Verification items for the finished model (mm, model axes). A direction names the side the tool comes from. Round coordinates to 2 decimals unless told otherwise and drop trailing zeros. Order: outer loops, then holes, each group sorted by start corner. A loop starts at its lowest first (then second) coordinate and runs counter-clockwise, first axis right, second up. Notation, with made-up numbers: (36, -21) -> (49, -21) arc R23 ccw to (49, -5) -> close; hole circle Ø7 at (-4.5, 39). An arc over 180 degrees is marked (long way). Return JSON: item names as keys, results as strings. Group by question number.
1) Draft check along Y on faces 1 (the cylindrical face through (64.305, 26.799, -2.273)), 2 (the flat face through (32, 7, -12)), 3 (the cylindrical face through (64.305, 48.012, -23.486)), 4 (the flat face through (78, 36, -11)). Enter one of: pulls with the +Y half, pulls with the -Y half, needs draft (parallel to the pull), parting line crosses it, or undercut.
2) Scan lines: L1, parallel to Z at x = 29, y = 33.5 (3 decimals); L2, parallel to Z at x = 29, y = 18 (3 decimals); L3, parallel to X at y = 18, z = 12.25 (3 decimals). Record each from-to range of solid material in increasing order.
3) Tool access check on faces 5 (the flat face through (51, 60, -35)), 6 (the cylindrical face through (32.5, 33.13, -44.32)). Record the directions out of +Z, -Z, +X, -X, +Y, -Y that give a thin tool (end or side, any length) a straight path to the whole face; none if there is none.
4) Section check A-A on y = 11. Enter the section's corners in (x, z) (3 decimals), plus the area to 3 significant figures.
5) Section check C-C on y = 23. State how many separate pieces and enclosed holes the cut face has, plus the area to 3 significant figures.
6) Depth check by flat-ended pin: pin 1 (6 mm diameter, centred on x = 40, y = 31, fed in from +Z); pin 2 (5 mm diameter, centred on x = 29, z = -35.75, fed in from -Y); pin 3 (5 mm diameter, centred on x = 60.5, z = -8.5, fed in from -Y); pin 4 (8 mm diameter, centred on y = 32, z = -37, fed in from +X). Enter the tip coordinate at first touch or a pass-through.
Solid Edge part; units mm, degrees
sketch "Sketch1" plane through (0, 0, 0) normal (0, -1, 0) x (1, 0, 0)
  line L0 (-34, -45.75) -> (34, -45.75)
  line L1 (34, -45.75) -> (34, 45.75)
  line L2 (34, 45.75) -> (-34, 45.75)
  line L3 (-34, 45.75) -> (-34, -45.75)
  dimension "D1" = 34
  dimension "D2" = 34
extrude "Protrusion1" add sketch "Sketch1" against normal blind 12
sketch "Sketch2" plane through (0, 0, 0) normal (0, -1, 0) x (1, 0, 0)
  circle A0 centre (0, -14.75) radius 11.25
  circle A1 centre (-15.5, 0.75) radius 1.7
  circle A2 centre (-15.5, -30.25) radius 1.7
  circle A3 centre (15.5, -30.25) radius 1.7
  circle A4 centre (15.5, 0.75) radius 1.7
extrude "Cutout1" cut sketch "Sketch2" against normal through all
sketch "Sketch3" plane through (0, 0, 0) normal (0, -1, 0) x (1, 0, 0)
  circle A0 centre (7.7782, 36.0282) radius 1.4
  circle A1 centre (7.7782, 20.4718) radius 1.4
  circle A2 centre (-7.7782, 20.4718) radius 1.4
  circle A3 centre (-7.7782, 36.0282) radius 1.4
  circle A4 centre (0, 28.25) radius 6
  dimension "D1" = 7.7782
extrude "Cutout2" cut sketch "Sketch3" against normal through all
sketch "Sketch4" plane through (-34, 6, 0) normal (-1, 0, 0) x (0, 0, -1)
  line L0 (-19.89, -6) -> (45.75, -71.64)
  line L1 (45.75, -71.64) -> (45.75, -6)
  line L2 (45.75, -6) -> (-19.89, -6)
extrude "Extrusionsausprägung_2" add sketch "Sketch4" against normal blind 10
mirror "Mirror1" about plane through (0, 0, 0) normal (1, 0, 0) of "Extrusionsausprägung_2"
sketch "Sketch5" plane through (-34, 38.82, 0) normal (-1, 0, 0) x (0, 0, -1)
  circle A0 centre (33.7465, 1.4635) radius 1.875
  circle A1 centre (19.6043, 15.6057) radius 1.875
  dimension "D1" = 19.6043
extrude "Extrusionsausschnitt_3" cut sketch "Sketch5" against normal blind 14
sketch "Sketch6" plane through (-34, 38.82, 0) normal (-1, 0, 0) x (0, 0, -1)
  line L0 (45.75, -38.82) -> (-31.89, 38.82)
  line L1 (-31.89, 38.82) -> (-17.75, 38.82)
  line L2 (-17.75, 38.82) -> (45.75, -24.68)
  line L3 (45.75, -24.68) -> (45.75, -38.82)
  dimension "D1" = 31.89
extrude "Extrusionsausprägung_4" add sketch "Sketch6" along normal blind 44
mirror "Mirror2" about plane through (0, 0, 0) normal (1, 0, 0) of "Extrusionsausprägung_4"
sketch "Sketch7" plane through (-54, 31.75, -14) normal (0, -0.7071, -0.7071) x (1, 0, 0)
  circle A0 centre (-14, 10.2613) radius 4
  circle A1 centre (-14, -19.7387) radius 4
extrude "Cutout3" cut sketch "Sketch7" against normal up to next
mirror "Mirror3" about plane through (0, 0, 0) normal (1, 0, 0) of "Cutout3"
sketch "Sketch8" plane through (-78, 38.82, -6.93) normal (-1, 0, 0) x (0, 0.7071, -0.7071)
  line L0 (29.953, 0) -> (42.4264, 12.4734)
extrude "Cutout4" cut sketch "Sketch8" against normal through all material side at (-78, 60.05, -36.93)
sketch "Sketch9" plane through (78, 30, -5.18) normal (1, 0, 0) x (0, -0.7071, 0.7071)
  line L0 (30.4551, -4.9992) -> (47.4257, -4.9992)
  line L1 (47.4257, -4.9992) -> (57.2262, -14.7997)
  line L2 (57.2262, -14.7997) -> (48.7409, -23.285)
  line L3 (48.7409, -23.285) -> (30.4551, -4.9992)
extrude "Extrusionsausschnitt_6" cut sketch "Sketch9" against normal blind 55
mirror "Mirror4" about plane through (0, 0, 0) normal (1, 0, 0) of "Extrusionsausschnitt_6"
fillet "Verrundung_1" radius 5 4 edges at (23, 6, 45.75) (-23, 6, 45.75) (34, 30, -45.75) (-34, 30, -45.75)
chamfer "Fase_1" distance 0.5 angle 45 2 edges at (-34, 23.2143, -17.7293) (-34, 37.3565, -31.8715)
chamfer "Fase_2" distance 0.4 angle 45 4 edges at (-17.2, 0, -30.25) (-17.2, 0, 0.75) (13.8, 0, 0.75) (13.8, 0, -30.25)
chamfer "Fase_3" distance 0.4 angle 45 4 edges at (-9.1782, 0, 20.4718) (-9.1782, 0, 36.0282) (6.3782, 0, 36.0282) (6.3782, 0, 20.4718)
chamfer "Fase_4" distance 2.5 angle 45 2 edges at (-11.25, 0, -14.75) (0, 12, -3.5)
chamfer "Fase_5" distance 1.4 angle 45 2 edges at (-6, 0, 28.25) (0, 12, 34.25)
chamfer "Fase_7" distance 1 angle 45 4 edges at (-68, 34.3926, -2.5026) (-68, 55.6058, -23.7158) (68, 34.3926, -2.5026) (68, 55.6058, -23.7158)
sketch "Sketch10" plane through (-78, 30, -5.18) normal (-1, 0, 0) x (0, 0.7071, -0.7071)
  line L0 (-30.4551, -4.9992) -> (-20.4566, 4.9992)
extrude "Extrusionsausschnitt_8" cut sketch "Sketch10" against normal blind 44 material side at (-78, 11.95, 12.82)
mirror "Mirror5" about plane through (0, 0, 0) normal (1, 0, 0) of "Extrusionsausschnitt_8"
sketch "Sketch11" plane through (0, 30, -45.75) normal (0, 0, -1) x (1, 0, 0)
  line L0 (34, 18) -> (-24, 18)
  line L1 (-24, 18) -> (-24, -30)
  line L2 (-24, -30) -> (-78, -30)
  line L3 (-78, -30) -> (-78, 30)
  line L4 (-78, 30) -> (34, 30)
  line L5 (34, 30) -> (34, 18)
extrude "Cutout6" cut sketch "Sketch11" against normal through all
sketch "Sketch12" plane through (51, 12, -12.93) normal (0, -1, 0) x (1, 0, 0)
  circle A0 centre (-22, 25.18) radius 1.875
  circle A1 centre (-22, 1.18) radius 1.875
  circle A2 centre (-22, -22.82) radius 1.875
  dimension "D1" = 22
extrude "Cutout7" cut sketch "Sketch12" against normal through all
sketch "Sketch13" plane through (51, 12, -12.93) normal (0, -1, 0) x (1, 0, 0)
  arc A0 (-22, -32.82) -> (-17, -27.82) centre (-22, -27.82) ccw
  line L0 (-17, 18.68) -> (-17, -27.82)
  line L1 (-17, 32.82) -> (-17, 18.68)
  line L2 (-27, 32.82) -> (-17, 32.82)
  line L3 (-27, 32.82) -> (-27, -32.82)
  line L4 (-27, -32.82) -> (-22, -32.82)
extrude "Extrusionsausprägung_6" add sketch "Sketch13" along normal blind 5
sketch "Sketch14" plane through (29, 7, -12.93) normal (0, -1, 0) x (0, 0, 1)
  circle A0 centre (25.18, 0) radius 1.875
  circle A1 centre (1.18, 0) radius 1.875
  circle A2 centre (-22.82, 0) radius 1.875
extrude "Cutout8" cut sketch "Sketch14" against normal through all
chamfer "Fase_8" distance 0.5 angle 45 3 edges at (29, 7, 10.375) (29, 7, -13.625) (29, 7, -37.625)
chamfer "Fase_9" distance 0.7 angle 45 2 edges at (72, 24.4942, -6.7442) (72, 45.7074, -27.9574)
properties material "Nylon, allgemein"
Check result:
{
 "1": {"face 1": "undercut", "face 2": "pulls with the -Y half", "face 3": "undercut", "face 4": "needs draft"},
 "2": {"L1": "-45.75 to -37.625, -33.875 to -13.625, -9.875 to -1.61", "L2": "-45.75 to -37.625, -33.875 to -13.625, -9.875 to 10.375", "L3": "24 to 27.125, 30.875 to 78"},
 "3": {"face 5": "+Z, -Z, +X, -X, +Y", "face 6": "-Z, +X, -Y"},
 "4": {"outline": "(24, -45.75) -> (29, -45.75) arc R5 ccw to (34, -40.75) -> (34, 19.89) -> (24, 19.89) -> close; hole circle Ø3.75 at (29, -35.75); hole circle Ø3.75 at (29, -11.75); hole circle Ø3.75 at (29, 12.25)", "area": "618 mm^2"},
 "5": {"separate pieces": "1", "enclosed holes": "2", "area": "1,130 mm^2"},
 "6": {"pin 1": "z = 3.89", "pin 2": "y = 7", "pin 3": "y = 23.75", "pin 4": "x = 34"}
}
